from build123d import *

# Parameters (mm, degrees)
F1_DEPTH = 7.112
F2_R     = 3.0734


with BuildPart() as f1:
    # F0 (on Front) → F1 (new body)
    with BuildSketch(Plane.XZ):
        with BuildLine():
            ThreePointArc((-4.623045, -4.602544), (0.345085, 0.365587), (5.313216, -4.602544))
            Line((5.313216, -4.602544), (5.313216, 5.577769))
            ThreePointArc((5.313216, 5.577769), (0.345085, 10.5459), (-4.623045, 5.577769))
            Line((-4.623045, 5.577769), (-4.623045, 2.380263))
            Line((-4.623045, 2.380263), (-4.623045, -4.602544))
        make_face()
        with BuildLine():
            ThreePointArc((-4.623045, -4.602544), (0.345085, -9.570675), (5.313216, -4.602544))
            Line((5.313216, -4.602544), (-4.623045, -4.602544))
        make_face()
        with BuildLine():
            Line((-4.623045, -4.602544), (5.313216, -4.602544))
            ThreePointArc((5.313216, -4.602544), (0.345085, 0.365587), (-4.623045, -4.602544))
        make_face()
        with BuildLine():
            ThreePointArc((-4.623045, -23.500242), (0.345085, -28.468372), (5.313216, -23.500242))
            Line((5.313216, -23.500242), (5.313216, -4.602544))
            ThreePointArc((5.313216, -4.602544), (0.345085, -9.570675), (-4.623045, -4.602544))
            Line((-4.623045, -4.602544), (-4.623045, -23.500242))
        make_face()
    extrude(amount=F1_DEPTH)

    # F2
    f2_edges = [f1.edges().sort_by_distance(p)[0] for p in [
        (5.313216, -7.112, -8.961236),
        (5.313216, 0, -8.961236),
        (0.345085, -7.112, 10.5459),
        (0.345085, 0, 10.5459),
        (0.345085, -7.112, -28.468372),
        (-4.623045, 0, -8.961236),
        (-4.623045, -7.112, -8.961236),
    ]]
    fillet(f2_edges, radius=F2_R)


solid = f1.part
Source: CAD feature listing. Evaluate the final solid. Frame: model axes, mm. Round coordinates to 2 decimals unless told otherwise and drop trailing zeros. Loops run counter-clockwise (first coordinate to the right, second up) from the corner with the lowest first, then second, coordinate; pieces in that order, holes last. Notation, with made-up numbers: (49.5, 30) - (98.5, 30) arc R20 ccw to (98.5, 47) - close; hole circle Ø5 at (34.25, 78.25). An arc over 180 degrees is marked (long way). Write item = value, one per line. Start each with the question number.
Item 1: Material intervals for line 1 (Y direction, x = 0, z = -25.5); line 2 (Y direction, x = 3.75, z = -23.5); line 3 (Z direction, x = 3.25, y = -2.25), sorted ascending.
Item 2: Section query A-A on z = -14. Output: boundary loops of the cut face in (x, y), plus the area to 3 significant figures.
Item 3: First-contact query: pin 1 Ø1 at (x, y) = (-2, -2) entering from +Z; pin 2 Ø4 at (y, z) = (-6.5, 3.5) entering from -X. Flat tips, straight axial feed; report the tip coordinate or a pass-through.
Results list:
q1.line_1 = -7.11 to 0
q1.line_2 = -6.72 to -0.4
q1.line_3 = -27.39 to 9.47
q2.outline = (-4.62, -4.04) arc R3.07 ccw to (-1.55, -7.11) - (2.24, -7.11) arc R3.07 ccw to (5.31, -4.04) - (5.31, -3.07) arc R3.07 ccw to (2.24, 0) - (-1.55, 0) arc R3.07 ccw to (-4.62, -3.07) - close
q2.area = 62.6 mm²
q3.pin_1 = 10.04
q3.pin_2 = -4.59
